from build123d import *

# Parameters (mm, degrees)
F1_DEPTH   = 120
F4_D       = 10
F4_ON_F3_D = 10
F6_D       = 10
F8_D       = 10


with BuildPart() as f1:
    # F0 (on Right) → F1 (new body)
    with BuildSketch(Plane.YZ):
        Polygon((0, 5), (0, 0), (60, 0), (60, 60), (55, 60), (55, 5), align=None)
    extrude(amount=F1_DEPTH)

    # F4 (through all)
    with Locations(Plane.XY.offset(5)):
        with Locations((46, 20), (19, 35)):
            Hole(F4_D / 2)

    # F4 on F3 (through all)
    with Locations(Plane.XZ.offset(-55)):
        with Locations((46, 40), (19, 25)):
            Hole(F4_ON_F3_D / 2)

    # F6 (through all)
    with Locations(Plane.XZ.offset(-55)):
        with Locations((100, 35)):
            Hole(F6_D / 2)

    # F8 (through all)
    with Locations(Plane.XY.offset(5)):
        with Locations((100, 25)):
            Hole(F8_D / 2)


solid = f1.part
CAD build for the part. Positions are in the model's coordinates, mm. A direction names the side the tool comes from. Give positions to 0.01 mm unless a question says otherwise; leave off trailing zeros. Write each loop counter-clockwise with the first axis right and the second up, starting at its lowest first coordinate (ties: lowest second). Pieces come first, ordered by that corner, then holes. Notation, with made-up numbers: M 50,51.5 L 66,51.5 A22 ccw 66,82.5 Z; hole C 9.5,88 d8. An arc over 180 degrees is marked long. Put each result on its own line as item: value. Start each with the question number.
(1) Band-saw the part on B-B, the plane x = 49. Write the cut outline in (y, z).
(2) Flat gauge pins, fed straight in: pin 1 Ø6 at (x, y) = (60, 36.5) entering from -Z; pin 2 Ø16 at (x, y) = (100, 25) entering from +Z; pin 3 Ø6 at (x, z) = (34.5, 49) entering from -Y; pin 4 Ø9 at (x, z) = (46, 40) entering from -Y. Where does each tip first touch, or does it go through?
(3) Mould opens along X. For faces 1 (the face through (120, 43, 3)), 2 (the face through (0, 43, 3)), 3 (the face through (20.08, 57.54, 20.12)) say: +X half, -X half, draft (parallel to the pull), parting line (faces both ways), or undercut.
(4) Probe L1, parallel to Y at x = 100, z = 3; L2, parallel to Y at x = 46, z = 2.95; L3, parallel to Z at x = 8, y = 15. List the from-to ranges inside material, lowest first.
(5) Band-saw the part on D-D, the plane x = 100. Write the cut outline in (y, z).
(6) Band-saw the part on C-C, the plane z = 25. Write the cut outline in (x, y).
(7) Which spindle directions (+Z, -Z, +X, -X, +Y, -Y) get a long thin tool onto all of the face, cutting with end or side? Do faces 4 (the face through (59, 58, 60)), 5 (the face through (59, 55, 33)). Say none if no direction does.
(8) Band-saw the part on A-A, the plane y = 17. Write the cut outline in (x, z).
Response values:
1. outline: M 0,0 L 16,0 L 16,5 L 0,5 Z; M 24,0 L 60,0 L 60,36 L 55,36 L 55,5 L 24,5 Z; M 55,44 L 60,44 L 60,60 L 55,60 Z
2. pin 1: stops at z = 0
2. pin 2: stops at z = 5
2. pin 3: stops at y = 55
2. pin 4: passes through
3. face 1: +X half
3. face 2: -X half
3. face 3: undercut
4. L1: y = 0 to 20, 30 to 60
4. L2: y = 0 to 15, 25 to 60
4. L3: z = 0 to 5
5. outline: M 0,0 L 20,0 L 20,5 L 0,5 Z; M 30,0 L 60,0 L 60,30 L 55,30 L 55,5 L 30,5 Z; M 55,40 L 60,40 L 60,60 L 55,60 Z
6. outline: M 0,55 L 14,55 L 14,60 L 0,60 Z; M 24,55 L 120,55 L 120,60 L 24,60 Z
7. face 4: +Z, +X, -X, +Y, -Y
7. face 5: +Z, +X, -X, -Y
8. outline: M 0,0 L 42,0 L 42,5 L 0,5 Z; M 50,0 L 120,0 L 120,5 L 50,5 Z
